from build123d import *

# Parameters (mm, degrees)
SKETCH_1_W          = 100
SKETCH_1_H          = 65
EXTRUDE_1_DEPTH     = 12
CUT_EXTRUDE_1_DEPTH = 10
SKETCH_2_3_R        = 3.5
CUT_EXTRUDE_2_DEPTH = 61.829680256
SKETCH_3_R          = 1.5
CUT_EXTRUDE_3_DEPTH = 10
CUT_EXTRUDE_START   = -10
SKETCH_4_R          = 1.5
CUT_EXTRUDE_4_DEPTH = 10
FILLET_2_R          = 4
FILLET_3_R          = 2


with BuildPart() as part:
    # 草图1 → 凸台-拉伸1 (new body)
    with BuildSketch(Plane.XY):
        Rectangle(SKETCH_1_W, SKETCH_1_H)
    extrude(amount=EXTRUDE_1_DEPTH)

    # 草图2 → 切除-拉伸1 (cut)
    with BuildSketch(Plane.XY.offset(12)):
        with BuildLine():
            Line((30, 31), (-30, 31))
            ThreePointArc((-30, 31), (-30.632455532, 30.897366596), (-31.2, 30.6))
            Line((-31.2, 30.6), (-32.8, 29.4))
            ThreePointArc((-32.8, 29.4), (-33.367544468, 29.102633404), (-34, 29))
            Line((-34, 29), (-41, 29))
            ThreePointArc((-41, 29), (-43.828427125, 27.828427125), (-45, 25))
            Line((-45, 25), (-45, 6))
            ThreePointArc((-45, 6), (-43.535533906, 2.464466094), (-40, 1))
            ThreePointArc((-40, 1), (-30, -9), (-40, -19))
            ThreePointArc((-40, -19), (-45, -24), (-40, -29))
            Line((-40, -29), (-34, -29))
            ThreePointArc((-34, -29), (-33.367544468, -29.102633404), (-32.8, -29.4))
            Line((-32.8, -29.4), (-31.2, -30.6))
            ThreePointArc((-31.2, -30.6), (-30.632455532, -30.897366596), (-30, -31))
            Line((-30, -31), (30, -31))
            ThreePointArc((30, -31), (30.632455532, -30.897366596), (31.2, -30.6))
            Line((31.2, -30.6), (32.8, -29.4))
            ThreePointArc((32.8, -29.4), (33.367544468, -29.102633404), (34, -29))
            Line((34, -29), (40, -29))
            ThreePointArc((40, -29), (45, -24), (40, -19))
            ThreePointArc((40, -19), (30, -9), (40, 1))
            ThreePointArc((40, 1), (43.535533906, 2.464466094), (45, 6))
            Line((45, 6), (45, 25))
            ThreePointArc((45, 25), (43.828427125, 27.828427125), (41, 29))
            Line((41, 29), (34, 29))
            ThreePointArc((34, 29), (33.367544468, 29.102633404), (32.8, 29.4))
            Line((32.8, 29.4), (31.2, 30.6))
            ThreePointArc((31.2, 30.6), (30.632455532, 30.897366596), (30, 31))
        make_face()
    extrude(amount=-CUT_EXTRUDE_1_DEPTH, mode=Mode.SUBTRACT)

    # 草图2<3> → 切除-拉伸2 (cut, through all)
    with BuildSketch(Plane.XY.offset(12)):
        with Locations((40, -9)):
            Circle(SKETCH_2_3_R)
        with Locations((-40, -9)):
            Circle(SKETCH_2_3_R)
    extrude(amount=-CUT_EXTRUDE_2_DEPTH, mode=Mode.SUBTRACT)

    # 草图3 → 切除-拉伸3 (cut)
    with BuildSketch(Plane(origin=(0, 32.5, 0), x_dir=(1, 0, 0), z_dir=(0, 1, 0))):
        with Locations(Location((40, -6, 0), (0, 0, 270))):
            Circle(SKETCH_3_R)
    cut_extrude_3 = extrude(amount=-CUT_EXTRUDE_3_DEPTH, mode=Mode.SUBTRACT)

    # 草图4 → 切除-拉伸4 (cut)
    with BuildSketch(Plane.XZ.offset(32.5).offset(CUT_EXTRUDE_START)):
        with Locations(Location((40, 6, 0), (0, 0, 90))):
            Circle(SKETCH_4_R)
    cut_extrude_4 = extrude(amount=CUT_EXTRUDE_4_DEPTH, mode=Mode.SUBTRACT)

    # 镜向1: 切除-拉伸3, 切除-拉伸4 across plane
    add(cut_extrude_3.mirror(Plane(origin=(0, 0, 0), x_dir=(0, 0, 1), z_dir=(1, 0, 0))), mode=Mode.SUBTRACT)
    add(cut_extrude_4.mirror(Plane(origin=(0, 0, 0), x_dir=(0, 0, 1), z_dir=(1, 0, 0))), mode=Mode.SUBTRACT)

    # 圆角2
    fillet_2_edges = [part.edges().sort_by_distance(p)[0] for p in [
        (-50, 0, 0),
        (50, 0, 0),
    ]]
    fillet(fillet_2_edges, radius=FILLET_2_R)

    # 圆角3
    fillet_3_edges = [part.edges().sort_by_distance(p)[0] for p in [
        (-50, 0, 12),
        (50, 0, 12),
    ]]
    fillet(fillet_3_edges, radius=FILLET_3_R)


solid = part.part
Could you check a few things on this model? Use its own coordinates, in mm. A direction names the side the tool comes from. Give positions to 0.01 mm unless a question says otherwise; leave off trailing zeros. Order: outer loops, then holes, each group sorted by start corner. A loop starts at its lowest first (then second) coordinate and runs counter-clockwise, first axis right, second up. Notation, with made-up numbers: (43, -12) - (63, -12) arc R24 cw to (63, 20) - close; hole circle Ø7 at (-22, 28). An arc over 180 degrees is marked (long way). One line per item, written item: value. Start each with the question number.
1. Thinking about a two-plate mould opening in Y: for faces 1 (the face through (30, -9, 7)), 2 (the face through (-43.797, 27.859, 7.07)), 3 (the face through (-50, 0, 7)), which applies, +Y half, -Y half, draft (parallel to the pull), parting line (faces both ways), or undercut?
2. For P1, Ø5, axis at x = -40, z = 6, coming from the -Y side; P2, Ø1.8, axis at x = 40, z = 6, coming from the +Y side; P3, Ø1, axis at x = 31, y = -0.5, coming from the +Z side; P4, Ø4, axis at x = 40, y = -9, coming from the -Z side, each with a flat end and sliding along its axis, tell me the tip position at first contact or that it passes through.
3. Imagine slicing it at B-B on z = 6. Give the number of separate pieces and of enclosed holes in the cut face, plus the area to 3 significant figures.
4. Imagine slicing it at C-C on x = 4. List the corners of the cut face in (y, z) for me, plus the area to 3 significant figures.
5. For faces 4 (the face through (-48.859, 0.455, 1.203)), 5 (the face through (45, -24, 7)), 6 (the face through (-38.536, 30.759, 5.675)), 7 (the face through (-41.464, -30.609, 5.675)), which set-ups out of +Z, -Z, +X, -X, +Y, -Y let a thin tool reach every point of the face, with its end or its side?
6. Imagine slicing it at A-A on y = -9. List the corners of the cut face in (x, z) for me.
7. If I drill on probe 1 along Y at (x, z) = (40, 10.5); probe 2 along X at (y, z) = (31.35, 6); probe 3 along Y at (x, z) = (-8, 4.25), over which ranges is the centre line in solid material (lowest first)?
8. Imagine slicing it at D-D on y = -24. List the corners of the cut face in (x, z) for me.
Values:
1. face 1: undercut
1. face 2: undercut
1. face 3: draft
2. P1: y = -32.5
2. P2: y = 1.08
2. P3: z = 2
2. P4: through
3. separate pieces: 4
3. enclosed holes: 2
3. area: 1,460 mm²
4. outline: (-32.5, 0) - (32.5, 0) - (32.5, 12) - (31, 12) - (31, 2) - (-31, 2) - (-31, 12) - (-32.5, 12) - close
4. area: 160 mm²
5. face 4: -Z, -X, +Y, -Y
5. face 5: +Z
5. face 6: +Y
5. face 7: -Y
6. outline: (-50, 4) arc R4 ccw to (-46, 0) - (-43.5, 0) - (-43.5, 12) - (-48, 12) arc R2 ccw to (-50, 10) - close; (-36.5, 0) - (36.5, 0) - (36.5, 12) - (30, 12) - (30, 2) - (-30, 2) - (-30, 12) - (-36.5, 12) - close; (43.5, 0) - (46, 0) arc R4 ccw to (50, 4) - (50, 10) arc R2 ccw to (48, 12) - (43.5, 12) - close
7. probe 1: -32.5 to -29, -19 to -12.5, -5.5 to 1, 29 to 32.5
7. probe 2: -50 to -41.5, -38.5 to 38.5, 41.5 to 50
7. probe 3: -32.5 to -31, 31 to 32.5
8. outline: (-50, 4) arc R4 ccw to (-46, 0) - (46, 0) arc R4 ccw to (50, 4) - (50, 10) arc R2 ccw to (48, 12) - (45, 12) - (45, 2) - (-45, 2) - (-45, 12) - (-48, 12) arc R2 ccw to (-50, 10) - close
